The model under review builds one solid part; all positions refer to its coordinate system, in mm. Round coordinates to 2 decimals unless told otherwise and drop trailing zeros. Order: outer loops, then holes, each group sorted by start corner. A loop starts at its lowest first (then second) coordinate and runs counter-clockwise, first axis right, second up. Notation, with made-up numbers: M 62.25,60 L 83.25,60 A24 ccw 83.25,73 Z; hole C 59,36 d5. An arc over 180 degrees is marked long. Answer as a JSON object with one key per item and string values. Group by question number.
1. Clearance check with flat-ended pins moving along their axes: P1, Ø3, axis at y = 10.5, z = 588.5, coming from the -X side; P2, Ø5.5, axis at x = -15, z = 762.5, coming from the +Y side; P3, Ø5, axis at y = 4, z = 229, coming from the -X side. State where each tip first meets the part, or that it passes through.
2. Add section A-A on z = 284. State the section outline as (x, y) points.
3. Add section B-B on y = 8.5. State the section outline as (x, z) points.
4. Mouldability with a two-part tool opening along Y and no side actions: class faces 1 (the face through (0, -15.634, 520)), 2 (the face through (-0.29, 17.36, 519.62)), 3 (the face through (0, -3, 1054)) as released by +Y, released by -Y, zero draft, split by the parting line, or undercut.
5. To check wall thickness, follow probe 1 along X at (y, z) = (-13.55, 1034); probe 2 along Z at (x, y) = (15, -11.65); probe 3 along X at (y, z) = (-5, 667.5). State the ranges of each line that lie inside material, in increasing order. Write a range as [from, to].
Autodesk Inventor part; units mm, degrees
ref_plane "YZ Plane" through (0, 0, 0) normal (1, 0, 0) x (0, 1, 0)
ref_plane "XZ Plane" through (0, 0, 0) normal (0, 1, 0) x (-1, 0, 0)
ref_plane "XY Plane" through (0, 0, 0) normal (0, 0, 1) x (1, 0, 0)
sketch "Esboço1" plane through (0, 0, 0) normal (0, 0, 1) x (1, 0, 0)
  arc A0 (4, 2.4377) -> (-4, 2.4377) centre (0, 9.3659) ccw
  line L0 (9.25, -3.9341) -> (9.25, -10.6341)
  line L1 (-9.25, -10.6341) -> (-9.25, -3.9341)
  line L2 (4, -15.6341) -> (-4, -15.6341)
  line L3 (20, -15.6341) -> (-20, -15.6341)
  line L4 (-20, -15.6341) -> (-20, -10.6341)
  line L5 (20, -10.6341) -> (20, -15.6341)
  line L6 (7.6788, -3.9341) -> (9.25, -3.9341)
  line L7 (-9.25, -3.9341) -> (-7.6788, -3.9341)
  line L8 (9.25, -10.6341) -> (20, -10.6341)
  line L9 (-20, -10.6341) -> (-9.25, -10.6341)
  line L10 (-4, 2.4377) -> (-7.6788, -3.9341)
  line L11 (-17.4151, -20.798) -> (-22.4188, -29.4646)
  line L12 (17.4151, -20.798) -> (23.6527, -31.6017)
  line L13 (9.25, -15.6341) -> (4, -15.6341)
  line L14 (0, -15.6341) -> (-9.25, -15.6341)
  line L15 (4, 2.4377) -> (7.6788, -3.9341)
  dimension "d6" = 16
  dimension "d7" = 25
  dimension "d8" = 18.5
  dimension "d9" = 11.7
  dimension "d10" = 8
  dimension "d13" = 5
  dimension "d14" = 40
extrude "Extrusão1" add sketch "Esboço1" along normal blind 1054
sketch "Esboço3" plane through (-20, -15.6341, 0) normal (0, -1, 0) x (1, 0, 0)
  line L0 (0, 1054) -> (40, 1054) construction
  line L1 (20, 1054) -> (20, 0) construction
  line L2 (20, 1034) -> (5, 1034) construction
  line L3 (5, 1034) -> (20, 1034) construction
  line L4 (20, 1034) -> (35, 1034) construction
  circle A0 centre (5, 1034) radius 2.75
  circle A1 centre (35, 1034) radius 2.75
  line L5 (40, 0) -> (0, 0) construction
  dimension "d18" = 15
  dimension "d19" = 15
  dimension "d20" = 5.5
  dimension "d21" = 5.5
  dimension "d22" = 20
hole "Furo1" at (-15, -15.6341, 1034) at (15, -15.6341, 1034) direction (0, 1, 0) diameter 5.5 depth 8 tip angle 118
properties part number "SBR16_EIXO_Y_2"
Recorded:
{
 "1": {"P1": "stops at x = -8", "P2": "stops at y = -10.63", "P3": "stops at x = -7.47"},
 "2": {"outline": "M -20,-15.63 L 20,-15.63 L 20,-10.63 L 9.25,-10.63 L 9.25,-3.93 L 7.68,-3.93 L 4,2.44 A8 ccw long -4,2.44 L -7.68,-3.93 L -9.25,-3.93 L -9.25,-10.63 L -20,-10.63 Z"},
 "3": {"outline": "M -7.95,0 L 7.95,0 L 7.95,1054 L -7.95,1054 Z"},
 "4": {"face 1": "released by -Y", "face 2": "undercut", "face 3": "zero draft"},
 "5": {"probe 1": "x = [-20, -17.75], [-12.25, 12.25], [17.75, 20]", "probe 2": "z = [0, 1031.25], [1036.75, 1054]", "probe 3": "x = [-9.25, 9.25]"}
}
